Work out the finished part from the listing and answer in its coordinate system (mm). A direction names the side the tool comes from. Coordinates: 2 decimals unless noted, no trailing zeros. Write each loop counter-clockwise with the first axis right and the second up, starting at its lowest first coordinate (ties: lowest second). Pieces come first, ordered by that corner, then holes. Notation, with made-up numbers: (76, 15.25) -> (107, 15.25) arc R16 ccw to (107, 41.25) -> close; hole circle Ø6 at (-26.5, 17). An arc over 180 degrees is marked (long way). Write each question's results on one line, items separated by ' | '. Start each with the question number.
from build123d import *

# Parameters (mm, degrees)
SKETCH_1_R          = 2
EXTRUDE_1_DEPTH     = 30
SKETCH_2_R          = 3
SKETCH_2_W          = 15
SKETCH_2_H          = 11
CUT_EXTRUDE_1_DEPTH = 44.647021662
CHAMFER_1_SIZE      = 3


with BuildPart() as part:
    # 草图1 → 凸台-拉伸1 (new, symmetric)
    with BuildSketch(Plane(origin=(0, 0, 0), x_dir=(0, 0, -1), z_dir=(1, 0, 0))):
        with BuildLine():
            Line((0, 0), (30, 0))
            Line((30, 0), (30, 4))
            Line((30, 4), (5, 4))
            ThreePointArc((5, 4), (-3.201562119, 9.126952648), (0, 0))
        make_face()
        with Locations((0, 5.125)):
            Circle(SKETCH_1_R, mode=Mode.SUBTRACT)
    extrude(amount=EXTRUDE_1_DEPTH, both=True)

    # 草图2 → 切除-拉伸1 (cut, through all)
    with BuildSketch(Plane(origin=(0, 0, 0), x_dir=(1, 0, 0), z_dir=(0, 1, 0))):
        with Locations(Location((-17, 18.5, 0), (0, 0, 90))):
            Circle(SKETCH_2_R)
        with Locations(Location((17, 18.5, 0), (0, 0, 90))):
            Circle(SKETCH_2_R)
        with Locations((22.5, 0.375)):
            Rectangle(SKETCH_2_W, SKETCH_2_H)
        with Locations((-22.5, 0.375)):
            Rectangle(SKETCH_2_W, SKETCH_2_H)
    extrude(amount=CUT_EXTRUDE_1_DEPTH, mode=Mode.SUBTRACT)

    # 倒角1
    chamfer_1_edges = [part.edges().sort_by_distance(p)[0] for p in [
        (22.5, 4, -5.875),
        (-22.5, 4, -5.875),
        (17, 4, -15.5),
        (-17, 4, -15.5),
        (0, 4, -30),
    ]]
    chamfer(chamfer_1_edges, length=CHAMFER_1_SIZE)


solid = part.part
1. Find section C-C on y = 5.75. Give the vertices of the cut face in (x, z).
2. Find section B-B on x = -17. Give the vertices of the cut face in (y, z) (3 decimals).
3. Find section A-A on z = -18.5. Give the vertices of the cut face in (x, y).
4. Find section D-D on x = 9. Give the vertices of the cut face in (y, z) (3 decimals), and give its area (3 significant figures).
5. Given pin 1 Ø5 at (x, y) = (-14, 1.5) entering from +Z; pin 2 Ø0.8 at (x, y) = (19, 0.5) entering from +Z (3 decimals); pin 3 Ø7 at (x, z) = (-17, -18.5) entering from +Y, each flat-ended and moving along its own axis, determine where each tip first touches the part or whether it passes through.
6. Find the intervals of material crossed by L1, parallel to X at y = 0.8, z = -18.5; L2, parallel to Y at x = 2, z = 0 (3 decimals); L3, parallel to Z at x = -17, y = 0.35 (3 decimals), in increasing order.
7. For faces 1 (the face through (22.605, 2.479, -7.354)), 2 (the face through (-15.2, 0.5, -16.1)), determine the directions among +Z, -Z, +X, -X, +Y, -Y from which every point of the face is accessible in a straight line to the end or side of a thin tool.
8. Determine the mould class of faces 3 (the face through (-30, 2, -18)), 4 (the face through (-0.21, 7.11, 0.26)), 5 (the face through (-22.395, 2.479, -7.354)) for opening direction Y: pulls with the +Y half, pulls with the -Y half, needs draft (parallel to the pull), parting line crosses it, or undercut.
Ans:
1) outline: (-15, -5.09) -> (15, -5.09) -> (15, -1.9) -> (-15, -1.9) -> close; (-15, 1.9) -> (15, 1.9) -> (15, 5.09) -> (-15, 5.09) -> close
2) outline: (0, -30) -> (1, -30) -> (4, -27) -> (4, -24.5) -> (1, -21.5) -> (0, -21.5) -> close; (0, -15.5) -> (1, -15.5) -> (4, -12.5) -> (4, -8.875) -> (1, -5.875) -> (0, -5.875) -> close
3) outline: (-30, 0) -> (-20, 0) -> (-20, 1) -> (-23, 4) -> (-30, 4) -> close; (-14, 0) -> (14, 0) -> (14, 1) -> (11, 4) -> (-11, 4) -> (-14, 1) -> close; (20, 0) -> (30, 0) -> (30, 4) -> (23, 4) -> (20, 1) -> close
4) outline: (0, -30) -> (1, -30) -> (4, -27) -> (4, -5) arc R5.125 ccw (long way) to (0, 0) -> close; hole circle Ø4 at (5.125, 0) | area: 171 mm²
5) pin 1: stops at z = 5 | pin 2: stops at z = -5.875 | pin 3: stops at y = 1.5
6) L1: x = -30 to -20, -14 to 14, 20 to 30 | L2: y = 0 to 3.125, 7.125 to 10.25 | L3: z = -30 to -21.5, -15.5 to -5.875
7) face 1: +Z, +X, +Y | face 2: +Y, -Y
8) face 3: needs draft | face 4: undercut | face 5: pulls with the +Y half
